Part model, mm, in its own coordinate system. A direction names the side the tool comes from. Coordinates: 2 decimals unless noted, no trailing zeros. Loops run counter-clockwise (first coordinate to the right, second up) from the corner with the lowest first, then second, coordinate; pieces in that order, holes last. Notation, with made-up numbers: (35.5, 52.25) - (80.5, 52.25) arc R12 ccw to (80.5, 75.25) - close; hole circle Ø10 at (54.25, 68.25). An arc over 180 degrees is marked (long way). Use a Markdown table: item, result. Add a question column.
1) Band-saw the part on B-B (x = 30). Give the cut face in (y, z), plus the area to 3 significant figures.
2) Drop flat-ended pins along their axis: P1, Ø9, axis at x = 27.5, y = 12.5, coming from the -Z side; P2, Ø1, axis at y = 7, z = -56.5, coming from the +X side; P3, Ø4, axis at x = 6.5, z = -28.5, coming from the -Y side; P4, Ø4, axis at y = 7, z = -16, coming from the +X side. Give the stop position or say it passes through.
3) Tool access for faces 1 (the face through (0, 9, -23)), 2 (the face through (30, 9, -28)), 3 (the face through (32.45, 8.87, -19.68)): list every direction of +Z, -Z, +X, -X, +Y, -Y with a clear straight run to the whole face (end or side of a thin tool).
4) Probe probe 1 along X at (y, z) = (5, -20); probe 2 along Z at (x, y) = (22, 9.5); probe 3 along X at (y, z) = (12.5, -10.5). List the from-to ranges inside material, lowest first. Write a range as [from, to].
5) Band-saw the part on A-A (z = -20). Give the cut face in (x, y).
6) Band-saw the part on C-C (z = -8.5). Give the cut face in (x, y), plus the area to 3 significant figures.
7) Pull direction X, two halves, no side cores. Call faces 4 (the face through (30, 9, 0)), 5 (the face through (60, 9, -22)), 6 (the face through (8, 9, -54)): +X half, -X half, draft (parallel to the pull), parting line (faces both ways), or undercut.
from build123d import *

# Parameters (mm, degrees)
BOSS_EXTRUDE1_DEPTH = 18
SKETCH3_R           = 2.469718116
CUT_EXTRUDE1_DEPTH  = 21


with BuildPart() as part:
    # Sketch1 → Boss-Extrude1 (new body)
    with BuildSketch(Plane(origin=(0, 0, 0), x_dir=(1, 0, 0), z_dir=(0, 1, 0))):
        with BuildLine():
            Line((8, 67.50149873), (8, 79.954057008))
            add(Edge.make_bspline(
                [(0, 45), (-4.267413412, 52.702157849), (-3.849710429, 67.232110416), (4.572220088, 77.524864833), (8, 79.954057008)],
                knots=[0, 0, 0, 0, 0.616858973, 0.90735247, 0.90735247, 0.90735247, 0.90735247], degree=3))
            Line((0, 45), (0, 28))
            Line((0, 28), (0, 0))
            Line((0, 0), (60, 0))
            Line((60, 0), (60, 28))
            Line((60, 28), (60, 45))
            add(Edge.make_bspline(
                [(60, 45), (64.267413412, 52.702157849), (63.849710429, 67.232110416), (55.427779912, 77.524864833), (52, 79.954057008)],
                knots=[0, 0, 0, 0, 0.616858973, 0.90735247, 0.90735247, 0.90735247, 0.90735247], degree=3))
            Line((52, 79.954057008), (52, 70.29729534))
            Line((52, 70.29729534), (52, 28))
            Line((52, 28), (8, 28))
            Line((8, 28), (8, 67.50149873))
        make_face()
    extrude(amount=BOSS_EXTRUDE1_DEPTH)

    # Sketch3 → Cut-Extrude1 (cut)
    with BuildSketch(Plane.XZ):
        with Locations(Location((30, -20, 0), (0, 0, 270))):
            Circle(SKETCH3_R)
    extrude(amount=-CUT_EXTRUDE1_DEPTH, mode=Mode.SUBTRACT)


solid = part.part
Answer block:
| question | item | result |
|---|---|---|
| 1 | outline | (0, -28) - (18, -28) - (18, -22.47) - (0, -22.47) - close; (0, -17.53) - (18, -17.53) - (18, 0) - (0, 0) - close |
| 1 | area | 415 mm2 |
| 2 | P1 | z = -28 |
| 2 | P2 | x = 63.09 |
| 2 | P3 | y = 0 |
| 2 | P4 | x = 60 |
| 3 | face 1 | +Z, -X, +Y, -Y |
| 3 | face 2 | -Z, +Y, -Y |
| 3 | face 3 | +Y, -Y |
| 4 | probe 1 | [0, 27.53], [32.47, 60] |
| 4 | probe 2 | [-28, 0] |
| 4 | probe 3 | [0, 60] |
| 5 | outline | (0, 0) - (27.53, 0) - (27.53, 18) - (0, 18) - close; (32.47, 0) - (60, 0) - (60, 18) - (32.47, 18) - close |
| 6 | outline | (0, 0) - (60, 0) - (60, 18) - (0, 18) - close |
| 6 | area | 1,080 mm2 |
| 7 | face 4 | draft |
| 7 | face 5 | +X half |
| 7 | face 6 | undercut |
